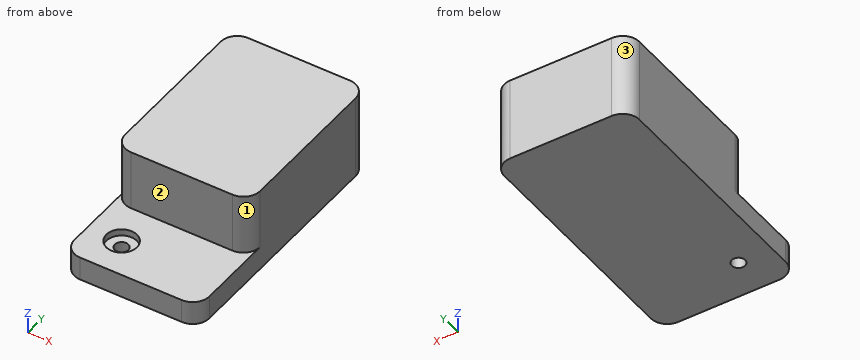
from build123d import *

# Parameters (mm, degrees)
F1_DEPTH = 127
F3_R     = 6.35
F4_DEPTH = 22.353
F2_R     = 14.396011
F5_DEPTH = 6.35
F6_R     = 15.748


with BuildPart() as f1:
    # F0 (on Right) → F1 (new body)
    with BuildSketch(Plane.YZ):
        Polygon((0, 22.352), (0, 0), (241.3, 0), (241.3, 79.502), (72.898, 79.502), (72.898, 22.352), align=None)
    extrude(amount=F1_DEPTH)

    # F3 (on face) → F4 (cut, through all)
    with BuildSketch(Plane.XY.offset(22.352)):
        with Locations((31.75, 35.052)):
            Circle(F3_R)
    extrude(amount=-F4_DEPTH, mode=Mode.SUBTRACT)

    # F2 (on face) → F5 (cut)
    with BuildSketch(Plane.XY.offset(22.352)):
        with Locations((31.75, 35.052)):
            Circle(F2_R)
    extrude(amount=-F5_DEPTH, mode=Mode.SUBTRACT)

    # F6
    f6_edges = [f1.edges().sort_by_distance(p)[0] for p in [
        (127, 72.898, 50.927),
        (127, 0, 11.176),
        (0, 0, 11.176),
        (0, 72.898, 50.927),
        (0, 241.3, 39.751),
        (127, 241.3, 39.751),
    ]]
    fillet(f6_edges, radius=F6_R)


solid = f1.part
The listing builds one solid part. Answer for the finished solid, in the listing's coordinates (mm). Face numbers are marked on the shaded views. A direction names the side the tool comes from. Round coordinates to 2 decimals unless told otherwise and drop trailing zeros. Write each loop counter-clockwise with the first axis right and the second up, starting at its lowest first coordinate (ties: lowest second). Pieces come first, ordered by that corner, then holes. Notation, with made-up numbers: M -30.75,36.5 L -23.75,36.5 A15 cw -23.75,41.5 Z; hole C 11.5,-19 d7. An arc over 180 degrees is marked long. Write each question's results on one line, items separated by ' | '. Start each with the question number.
Item 1: Find section A-A on x = 31.75. Write down the section's boundary in (y, z), and give its area (3 significant figures).
Item 2: Straight lines are drawn through the part: probe 1 along Y at (x, z) = (31, 3); probe 2 along Y at (x, z) = (31.75, 18.25); probe 3 along Z at (x, y) = (114, 50). For each, find the intervals that lie inside material, in ascending order.
Item 3: Given pin 1 Ø14.5 at (x, y) = (31.75, 35.052) entering from +Z; pin 2 Ø1.5 at (y, z) = (71, 71) entering from +X; pin 3 Ø8 at (x, z) = (50, 69.5) entering from -Y, each flat-ended and moving along its own axis, determine where each tip first touches the part or whether it passes through.
Item 4: Find section C-C on z = 63. Write down the section's boundary in (x, y), and give its area (3 significant figures).
Item 5: Find section D-D on x = 13. Write down the section's boundary in (y, z).
Item 6: Which of the six approach directions +Z, -Z, +X, -X, +Y, -Y give full straight-line access (tool end or side, diameter ignored) to the marked faces 1, 2 and 3?
Item 7: Find section B-B on x = 62. Write down the section's boundary in (y, z).
Answer block:
1) outline: M 0,0 L 28.7,0 L 28.7,16 L 20.66,16 L 20.66,22.35 L 0,22.35 Z; M 41.4,0 L 241.3,0 L 241.3,79.5 L 72.9,79.5 L 72.9,22.35 L 49.45,22.35 L 49.45,16 L 41.4,16 Z | area: 14,600 mm²
2) probe 1: y = 0 to 28.75, 41.36 to 241.3 | probe 2: y = 0 to 20.66, 49.45 to 241.3 | probe 3: z = 0 to 22.35
3) pin 1: stops at z = 16 | pin 2: passes through | pin 3: stops at y = 72.9
4) outline: M 0,88.65 A15.75 ccw 15.75,72.9 L 111.25,72.9 A15.75 ccw 127,88.65 L 127,225.55 A15.75 ccw 111.25,241.3 L 15.75,241.3 A15.75 ccw 0,225.55 Z | area: 21,200 mm²
5) outline: M 0.24,0 L 241.06,0 L 241.06,79.5 L 73.14,79.5 L 73.14,22.35 L 0.24,22.35 Z
6) face 1: +Z, +X, -Y | face 2: +Z, +X, -X, -Y | face 3: +Z, -Z, -X, +Y
7) outline: M 0,0 L 241.3,0 L 241.3,79.5 L 72.9,79.5 L 72.9,22.35 L 0,22.35 Z
